from build123d import *

# Parameters (mm, degrees)
HEAD_DEPTH         = 4
SHANK_SKETCH_R     = 2
SHANK_DEPTH        = 25
SKETCH6_R          = 2.625
HEAD_CUT_DEPTH     = 1
FILLET1_R          = 1
SKETCH7_W          = 3.5
SKETCH7_H          = 0.5
CUT_EXTRUDE1_DEPTH = 1


with BuildPart() as part:
    # Head Sketch → Head (new body)
    with BuildSketch(Plane.XY):
        Polygon((0, 4.041451884), (3.5, 2.020725942), (3.5, -2.020725942), (0, -4.041451884), (-3.5, -2.020725942), (-3.5, 2.020725942), align=None)
    extrude(amount=HEAD_DEPTH)

    # Shank Sketch → Shank (add)
    with BuildSketch(Plane.XY):
        Circle(SHANK_SKETCH_R)
    extrude(amount=-SHANK_DEPTH)

    # Sketch3 → Flange (revolve)
    with BuildSketch(Plane(origin=(0, 0, 0), x_dir=(-1, 0, 0), z_dir=(0, 1, 0)), mode=Mode.PRIVATE) as flange_sk:
        with BuildLine():
            Line((-5, 0), (0, 0))
            Line((0, 0), (0, 1.5))
            ThreePointArc((0, 1.5), (-2.562220765, 1.372207648), (-5.099009901, 0.99009901))
            ThreePointArc((-5.099009901, 0.99009901), (-5.497518595, 0.45024814), (-5, 0))
        make_face()
    revolve(flange_sk.sketch.rotate(Axis((0, 0, 0), (0, 0, 1)), 30), axis=Axis((0, 0, 0), (0, 0, 1)))

    # Sketch5 → Head Trim (revolve, cut)
    with BuildSketch(Plane(origin=(0, 0, 0), x_dir=(0, 0, -1), z_dir=(1, 0, 0)), mode=Mode.PRIVATE) as head_trim_sk:
        with BuildLine():
            Line((-4, -3.041451884), (-4, -4.041451884))
            Line((-4, -4.041451884), (-3, -4.041451884))
            ThreePointArc((-3, -4.041451884), (-3.707106781, -3.748558666), (-4, -3.041451884))
        make_face()
    revolve(head_trim_sk.sketch.rotate(Axis((0, 0, 15.085599173), (0, 0, -1)), 90), axis=Axis((0, 0, 15.085599173), (0, 0, -1)), mode=Mode.SUBTRACT)

    # Sketch6 → Head Cut (cut)
    with BuildSketch(Plane.XY.offset(4)):
        Circle(SKETCH6_R)
    extrude(amount=-HEAD_CUT_DEPTH, mode=Mode.SUBTRACT)

    # Fillet1
    fillet1_edges = [part.edges().sort_by_distance(p)[0] for p in [
        (-2.625, 0, 3),
    ]]
    fillet(fillet1_edges, radius=FILLET1_R - 0.0001)  # a hair under: the kernel refuses the full size

    # Sketch7 → Cut-Extrude1 (cut)
    with BuildSketch(Plane(origin=(0.741825606, 1.407208117, 4), x_dir=(1, 0, 0), z_dir=(0, 0, 1))):
        with Locations((1.008174394, -1.407208117)):
            Rectangle(SKETCH7_W, SKETCH7_H)
    extrude(amount=-CUT_EXTRUDE1_DEPTH, mode=Mode.SUBTRACT)


solid = part.part
CAD build for the part. Positions are in the model's coordinates, mm. A direction names the side the tool comes from. Round coordinates to 2 decimals unless told otherwise and drop trailing zeros. Write each loop counter-clockwise with the first axis right and the second up, starting at its lowest first coordinate (ties: lowest second). Pieces come first, ordered by that corner, then holes. Notation, with made-up numbers: (-8.75, 70) -> (40.25, 70) arc R19 cw to (40.25, 94) -> close; hole circle Ø5 at (11.25, -12). An arc over 180 degrees is marked (long way). Answer as a JSON object with one key per item and string values.
(1) Which spindle directions (+Z, -Z, +X, -X, +Y, -Y) get a long thin tool onto all of the face, cutting with end or side? Do faces 1 (the face through (3, 0.25, 3.4)), 2 (the face through (1.8, -3, 2.5)), 3 (the face through (1.725, 3.045, 2.516)), 4 (the face through (2, 1, 0)), 5 (the face through (-1.8, 3, 2.5)). Say none if no direction does.
Reported:
{"face 1": "+Z, +X", "face 2": "+Z, +X, -Y", "face 3": "+Z, +X, +Y", "face 4": "-Z", "face 5": "+Z, -X, +Y"}
(2) Probe probe 1 along Z at (x, y) = (-2.25, -2); probe 2 along X at (y, z) = (1, 1.5); probe 3 along Z at (x, y) = (0, -3.5). List the from-to ranges inside material, lowest first. Write a range as [from, to].
Reported:
{"probe 1": "z = [0, 4]", "probe 2": "x = [-3.5, 3.5]", "probe 3": "z = [0, 3.89]"}
(3) Pin check, flat tips, straight feed: P1, Ø2, axis at x = -0.5, y = -3.5, coming from the -Z side; P2, Ø1.1, axis at x = 2.5, z = 3.5, coming from the -Y side; P3, Ø2, axis at y = -0.5, z = 2.5, coming from the +X side. Stop position of each tip, or through.
Reported:
{"P1": "stops at z = 0", "P2": "stops at y = -2.92", "P3": "stops at x = 3.5"}
(4) Two-plate mould, pull along X, no slides. Class faces 6 (the face through (-1.725, -3.045, 2.516)), 7 (the face through (0, 0, 3)), 8 (the face through (0, 0, -25)): +X half, -X half, draft (parallel to the pull), parting line (faces both ways), or undercut.
Reported:
{"face 6": "-X half", "face 7": "undercut", "face 8": "draft"}
(5) Band-saw the part on A-A, the plane z = -2.5. List the corners of the cut face in (x, y), then the cut area to 3 significant figures.
Reported:
{"outline": "circle Ø4 at (0, 0)", "area": "12.6 mm^2"}
